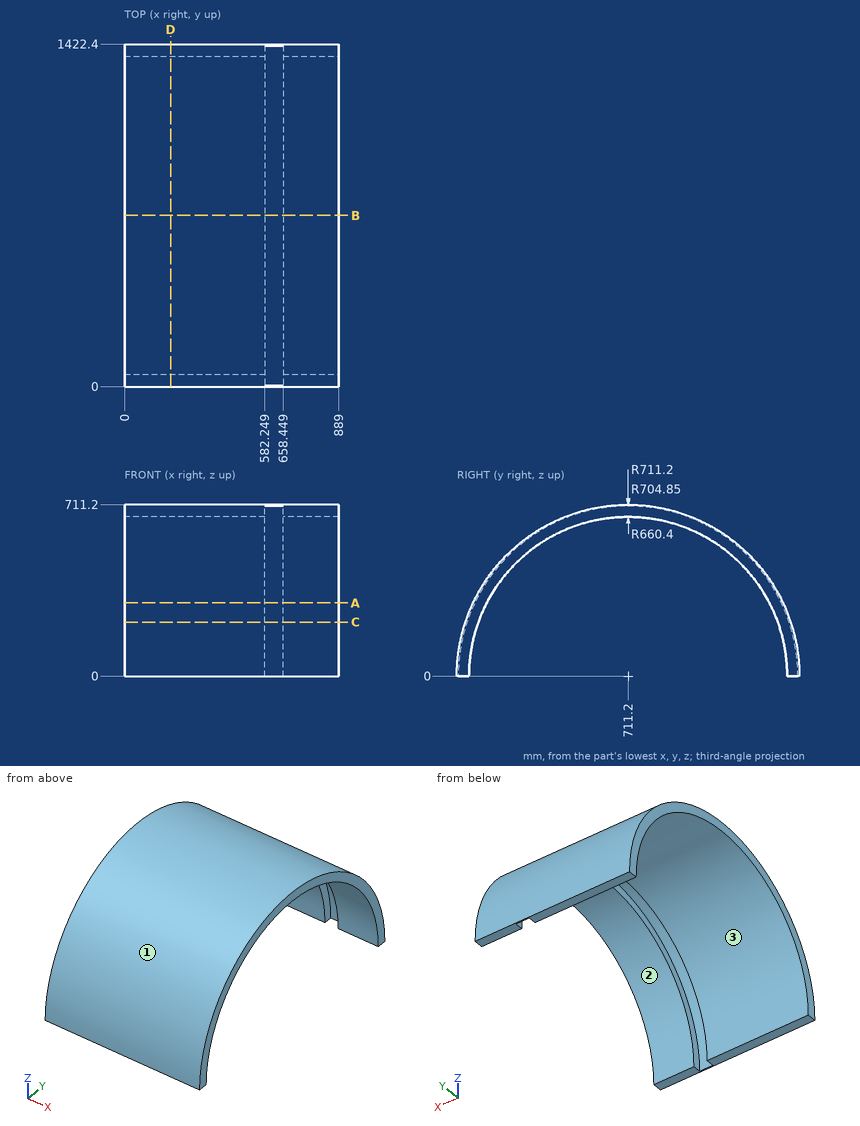
Design review of the part shown in the three views and the two pictorial views. Dimensions are in mm from the part's minimum x, y and z. Give positions to 0.01 mm unless a question says otherwise; leave off trailing zeros. Loops run counter-clockwise (first coordinate to the right, second up) from the corner with the lowest first, then second, coordinate; pieces in that order, holes last. Notation, with made-up numbers: M 45.5,43.5 L 94.5,43.5 A35 ccw 94.5,76.5 Z; hole C -10.5,49.25 d4. An arc over 180 degrees is marked long. Answer as a JSON object with one key per item and string values. Group by question number.
Q1. Add section C-C on z = 224. Give the boundary of the cut face in (x, y).
Q2. Insertion check: P1, Ø1.5, axis at x = 348.5, z = 638, coming from the -Y side; P2, Ø6, axis at x = 679, y = 861, coming from the -Z side; P3, Ø4, axis at x = 520.5, y = 698, coming from the +Z side. Each pin has a flat end and moves straight along its axis. Give the tip position at first contact, or say it passes through.
Q3. Mouldability with a two-part tool opening along Y and no side actions: class the marked faces 1, 2 and 3 as +Y half, -Y half, draft (parallel to the pull), parting line (faces both ways), or undercut.
Q4. For probe 1 along X at (y, z) = (1124, 526.5); probe 2 along Y at (x, z) = (831, 364.5); probe 3 along Y at (x, z) = (706.5, 360.5), list the stretches that pass through material, from the lowest coordinate up. Write a range as [from, to].
Q5. Add section A-A on z = 304. Give the boundary of the cut face in (x, y).
Q6. Add section B-B on y = 711.2. Give the boundary of the cut face in (x, z).
Q7. Add section D-D on x = 191.5. Give the boundary of the cut face in (y, z).
Checked values:
{
 "1": {"outline": "M 0,36.2 L 889,36.2 L 889,89.95 L 658.45,89.95 L 658.45,42.89 L 582.25,42.89 L 582.25,89.95 L 0,89.95 Z; M 0,1332.45 L 582.25,1332.45 L 582.25,1379.51 L 658.45,1379.51 L 658.45,1332.45 L 889,1332.45 L 889,1386.2 L 0,1386.2 Z"},
 "2": {"P1": "y = 395.42", "P2": "z = 642.48", "P3": "z = 711.11"},
 "3": {"face 1": "parting line", "face 2": "undercut", "face 3": "undercut"},
 "4": {"probe 1": "[0, 582.25], [658.45, 889]", "probe 2": "[100.51, 160.5], [1261.9, 1321.89]", "probe 3": "[98.14, 157.88], [1264.52, 1324.26]"},
 "5": {"outline": "M 0,68.25 L 889,68.25 L 889,124.93 L 658.45,124.93 L 658.45,75.28 L 582.25,75.28 L 582.25,124.93 L 0,124.93 Z; M 0,1297.47 L 582.25,1297.47 L 582.25,1347.12 L 658.45,1347.12 L 658.45,1297.47 L 889,1297.47 L 889,1354.15 L 0,1354.15 Z"},
 "6": {"outline": "M 0,660.4 L 582.25,660.4 L 582.25,704.85 L 658.45,704.85 L 658.45,660.4 L 889,660.4 L 889,711.2 L 0,711.2 Z"},
 "7": {"outline": "M 0,0 L 50.8,0 A660.4 cw 1371.6,0 L 1422.4,0 A711.2 ccw Z"}
}
